Here's the drawing with two shaded views (mm, measured from the low corner). I have some questions. A direction names the side the tool comes from. Give positions to 0.01 mm unless a question says otherwise; leave off trailing zeros. Loops run counter-clockwise (first coordinate to the right, second up) from the corner with the lowest first, then second, coordinate; pieces in that order, holes last. Notation, with made-up numbers: M 15,26.5 L 44,26.5 A24 ccw 44,46.5 Z; hole C -39,11 d5. An arc over 180 degrees is marked long. Write item = value, one per line. Start each with the question number.
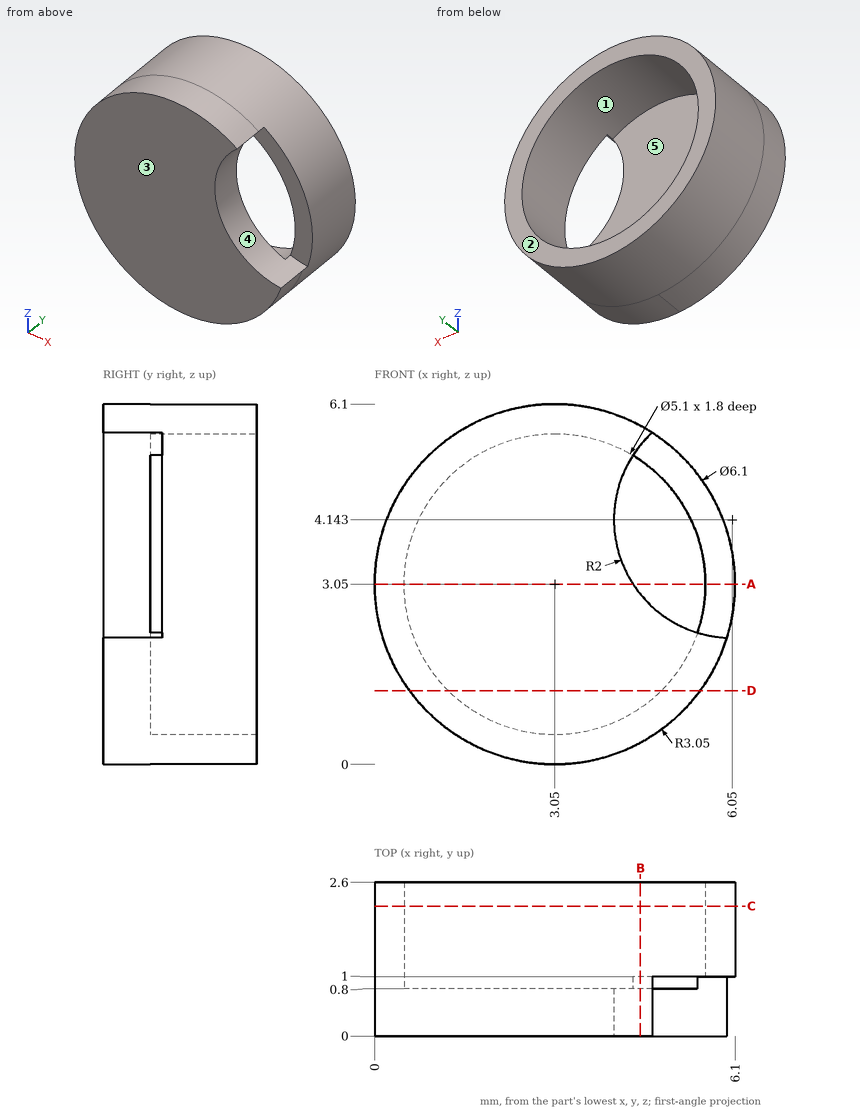
Q1. If we section it at A-A, the plane z = 3.05: List the corners of the cut face in (x, y) for me (1 decimal).
Q2. Will these pins go through, and if not, where does the flat tip stop? pin 1 (1.5 mm diameter, centred on x = 3, z = 3, fed in from +Y); pin 2 (1.9 mm diameter, centred on x = 5.5, z = 4.5, fed in from -Y).
Q3. If we section it at D-D, the plane z = 1.25: List the corners of the cut face in (x, y) for me.
Q4. If we section it at B-B, the plane x = 4.5: List the corners of the cut face in (y, z) for me.
Q5. On a 3-axis mill with a long thin cutter (end or side, diameter ignored), from which of +Z, -Z, +X, -X, +Y, -Y can I reach the whole of each face in a straight line? I mean the marked faces 1 and 2. Say none if no direction works.
Q6. We'd pull the mould along X, two halves only. Please class the marked faces 3, 4 and 5: pulls with the +X half, pulls with the -X half, needs draft (parallel to the pull), parting line crosses it, or undercut.
Q7. If we section it at C-C, the plane y = 2.2: List the corners of the cut face in (x, z) for me.
Q8. If I drill on line 1 along Z through (x, y) = (3, 2.1); line 2 along Y through (x, z) = (3.5, 0.75), over which ranges is the centre line in solid material (lowest first)?
Resolved:
q1.outline = M 0,0 L 4.4,0 L 4.4,0.8 L 0.5,0.8 L 0.5,2.6 L 0,2.6 Z; M 5.6,1 L 6.1,1 L 6.1,2.6 L 5.6,2.6 Z
q2.pin_1 = 0.8
q2.pin_2 = 1
q3.outline = M 0.59,0 L 5.51,0 L 5.51,2.6 L 4.86,2.6 L 4.86,0.8 L 1.24,0.8 L 1.24,2.6 L 0.59,2.6 Z
q4.outline = M 0,0.37 L 2.6,0.37 L 2.6,0.95 L 0.8,0.95 L 0.8,2.88 L 0,2.88 Z; M 0,5.41 L 1,5.41 L 1,5.15 L 2.6,5.15 L 2.6,5.73 L 0,5.73 Z
q5.face_1 = +Y
q5.face_2 = +Z, -Z, +X, -X, +Y
q6.face_3 = needs draft
q6.face_4 = pulls with the +X half
q6.face_5 = undercut
q7.outline = C 3.05,3.05 d6.1; hole C 3.05,3.05 d5.1
q8.line_1 = 0 to 0.5, 5.6 to 6.1
q8.line_2 = 0 to 0.8
